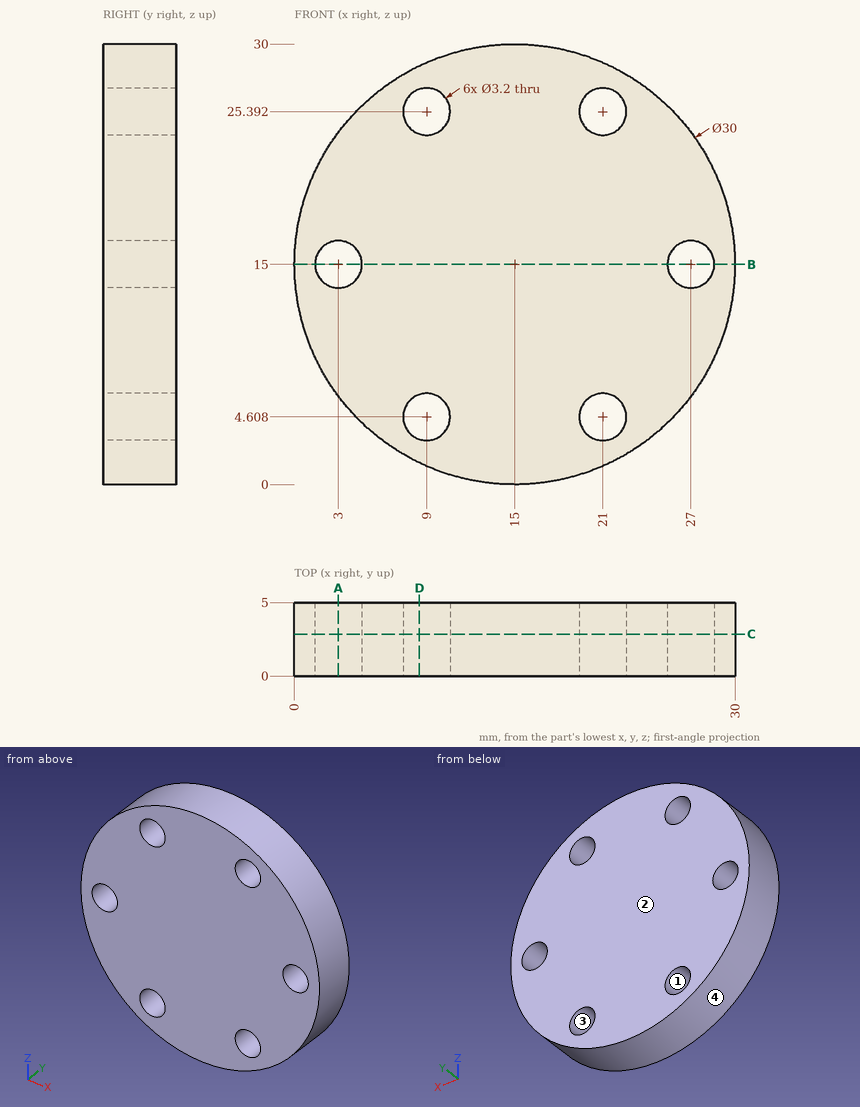
Study the drawing (mm; zero at the part's minimum x, y, z) and answer. Coordinates: 2 decimals unless noted, no trailing zeros. Order: outer loops, then holes, each group sorted by start corner. A loop starts at its lowest first (then second) coordinate and runs counter-clockwise, first axis right, second up. Notation, with made-up numbers: M 40.25,83 L 95.25,83 A22 ccw 95.25,115 Z; hole C -37.75,85 d11. An arc over 180 degrees is marked long. Answer as a JSON object with one key per item and string values. Group by question number.
1. Flat-ended cylindrical pins translate along their axes: P1, Ø2, axis at x = 8.5, z = 12.5, coming from the -Y side; P2, Ø2, axis at x = 4.5, y = 4, coming from the -Z side; P3, Ø2, axis at y = 1, z = 4, coming from the -X side; P4, Ø2.5, axis at x = 9, z = 25.39, coming from the -Y side. Find the tip coordinate at first contact, or state that the pin passes through.
2. Section D-D on x = 8.5 is taken. Write down the section's boundary in (y, z).
3. Determine the mould class of the marked faces 1, 2, 3 and 4 for opening direction Z: released by +Z, released by -Z, zero draft, split by the parting line, or undercut.
4. Straight lines are drawn through the part: line 1 (Z direction, x = 9, y = 2.2); line 2 (X direction, y = 2.9, z = 24.5); line 3 (X direction, y = 3.95, z = 4.25). For each, find the intervals that lie inside material, in ascending order.
5. Section C-C on y = 2.85 is taken. Write down the section's boundary in (x, z), then the cut area to 3 significant figures.
6. Section B-B on z = 15 is taken. Write down the section's boundary in (x, y).
7. Section A-A on x = 3 is taken. Write down the section's boundary in (y, z), then the cut area to 3 significant figures.
Values follow:
{
 "1": {"P1": "y = 0", "P2": "z = 3.39", "P3": "x = 3.82", "P4": "through"},
 "2": {"outline": "M 0,1.48 L 5,1.48 L 5,3.09 L 0,3.09 Z; M 0,6.13 L 5,6.13 L 5,23.87 L 0,23.87 Z; M 0,26.91 L 5,26.91 L 5,28.52 L 0,28.52 Z"},
 "3": {"face 1": "undercut", "face 2": "zero draft", "face 3": "undercut", "face 4": "split by the parting line"},
 "4": {"line 1": "1.25 to 3.01, 6.21 to 23.79, 26.99 to 28.75", "line 2": "3.39 to 7.67, 10.33 to 19.67, 22.33 to 26.61", "line 3": "4.54 to 7.44, 10.56 to 19.44, 22.56 to 25.46"},
 "5": {"outline": "C 15,15 d30; hole C 3,15 d3.2; hole C 9,4.61 d3.2; hole C 9,25.39 d3.2; hole C 21,4.61 d3.2; hole C 21,25.39 d3.2; hole C 27,15 d3.2", "area": "659 mm2"},
 "6": {"outline": "M 0,0 L 1.4,0 L 1.4,5 L 0,5 Z; M 4.6,0 L 25.4,0 L 25.4,5 L 4.6,5 Z; M 28.6,0 L 30,0 L 30,5 L 28.6,5 Z"},
 "7": {"outline": "M 0,6 L 5,6 L 5,13.4 L 0,13.4 Z; M 0,16.6 L 5,16.6 L 5,24 L 0,24 Z", "area": "74.0 mm2"}
}
